The model under review builds one solid part; all positions refer to its coordinate system, in mm. A direction names the side the tool comes from. Round coordinates to 2 decimals unless told otherwise and drop trailing zeros. Answer in a Markdown table with one row per item. Add a question column.
```python
from build123d import *

# Parameters (mm, degrees)
BOSS_EXTRUDE1_DEPTH = 40
BOSS_EXTRUDE3_DEPTH = 29.899298
SKETCH3_R           = 3
CUT_EXTRUDE1_DEPTH  = 30.899298
SKETCH4_R           = 3
CUT_EXTRUDE2_DEPTH  = 38.007847
FILLET1_R           = 3
CHAMFER1_SIZE       = 1


with BuildPart() as part:
    # Sketch1 → Boss-Extrude1 (new body)
    with BuildSketch(Plane.XY):
        Polygon((0, 15), (14.899298, 15), (14.899298, -14.949649), (-15, -14.949649), (-15, 15), align=None)
        Polygon((-9.966433, 9.966433), (-4.741433, 9.966433), (-3.1, 8.307461), (-5.5, 8.307461), (-5.5, 6.667461), (-2.79, 3.957461), (2.79, 3.957461), (5.5, 6.667461), (5.5, 8.307461), (3.1, 8.307461), (4.741433, 9.966433), (9.966433, 9.966433), (9.966433, 4.741433), (8.307461, 3.1), (8.307461, 5.5), (6.667461, 5.5), (3.957461, 2.79), (3.957461, -2.79), (6.667461, -5.5), (8.307461, -5.5), (8.307461, -3.1), (9.966433, -4.741433), (9.966433, -9.966433), (4.741433, -9.966433), (3.1, -8.307461), (5.5, -8.307461), (5.5, -6.667461), (2.79, -3.957461), (-2.79, -3.957461), (-5.5, -6.667461), (-5.5, -8.307461), (-3.1, -8.307461), (-4.741433, -9.966433), (-9.966433, -9.966433), (-9.966433, -4.741433), (-8.307461, -3.1), (-8.307461, -5.5), (-6.667461, -5.5), (-3.957461, -2.79), (-3.957461, 2.79), (-6.667461, 5.5), (-8.307461, 5.5), (-8.307461, 3.1), (-9.966433, 4.741433), align=None, mode=Mode.SUBTRACT)
    extrude(amount=BOSS_EXTRUDE1_DEPTH)

    # Sketch5 → Boss-Extrude3 (add, through all)
    with BuildSketch(Plane.ZY.offset(15)):
        with BuildLine():
            Line((0, 21.5), (0, 15))
            Line((0, 15), (12, 15))
            ThreePointArc((12, 15), (9.45049, 27.47913), (16.690416, 17))
            Line((16.690416, 17), (27.804488, 17))
            Line((27.804488, 17), (40, 17))
            Line((40, 17), (40, 21))
            Line((40, 21), (23.989579, 21))
            ThreePointArc((23.989579, 21), (12.250054, 33.497394), (0, 21.5))
        make_face()
    extrude(amount=-BOSS_EXTRUDE3_DEPTH)

    # Sketch3 → Cut-Extrude1 (cut, through all)
    with BuildSketch(Plane.ZY.offset(15)):
        with Locations((12, 0)):
            Circle(SKETCH3_R)
        with Locations((27, 0)):
            Circle(SKETCH3_R)
    extrude(amount=-CUT_EXTRUDE1_DEPTH, mode=Mode.SUBTRACT)

    # Sketch4 → Cut-Extrude2 (cut, through all)
    with BuildSketch(Plane(origin=(0, 22.058198, 0), x_dir=(1, 0, 0), z_dir=(0, 1, 0))):
        with Locations((0, -32.5)):
            Circle(SKETCH4_R)
    extrude(amount=-CUT_EXTRUDE2_DEPTH, mode=Mode.SUBTRACT)

    # Fillet1
    fillet1_edges = [part.edges().sort_by_distance(p)[0] for p in [
        (-0.050351, -14.949649, 40),
        (14.899298, 0.025175, 40),
        (14.899298, 33.497394, 12.250054),
        (14.899298, 21, 31.994789),
        (14.899298, 19, 40),
        (-0.050351, 21, 40),
        (-15, 19, 40),
        (-15, 21, 31.994789),
        (-15, 33.497394, 12.250054),
        (14.899298, 0.025175, 0),
        (-0.050351, -14.949649, 0),
        (-15, 3.275175, 0),
        (-15, 0.025175, 40),
        (14.899298, -14.949649, 20),
        (-15, -14.949649, 20),
    ]]
    fillet(fillet1_edges, radius=FILLET1_R)

    # Chamfer1
    chamfer1_edges = [part.edges().sort_by_distance(p)[0] for p in [
        (14.899298, 0, 9),
        (-15, 0, 9),
        (14.899298, 0, 24),
        (-15, 0, 24),
        (-3, -14.949649, 32.5),
        (-3, 21, 32.5),
    ]]
    chamfer(chamfer1_edges, length=CHAMFER1_SIZE)


solid = part.part
```
1. Tool access review of faces 4 (the cylindrical face through (-14.14, 1.71, 39.1)), 5 (the flat face through (5.5, -7, 20)), 6 (the flat face through (0, 17, 28)): name each direction out of +Z, -Z, +X, -X, +Y, -Y from which nothing blocks a thin tool from reaching the whole face with its end or side.
2. For L1, parallel to Z at x = -11.5, y = 0; L2, parallel to Y at x = -10.5, z = 12; L3, parallel to Y at x = -6.75, z = 12, list the stretches that pass through material, from the lowest coordinate up.
3. Add section A-A on x = 0. State how many separate pieces and enclosed holes the cut face has, plus the area to 3 significant figures.
4. Mouldability with a two-part tool opening along X and no side actions: class faces 1 (the flat face through (0, 9, 0)), 2 (the cylindrical face through (-0.65, 18.52, 35.43)), 3 (the cylindrical face through (14.04, 20.1, 30.39)) as pulls with the +X half, pulls with the -X half, needs draft (parallel to the pull), parting line crosses it, or undercut.
5. Insertion check: pin 1 Ø5 at (y, z) = (22, 32.5) entering from -X; pin 2 Ø5.5 at (y, z) = (0, 27) entering from +X; pin 3 Ø5.5 at (x, z) = (-7, 21) entering from +Y; pin 4 Ø8 at (x, z) = (7.5, 9) entering from +Y. Each pin has a flat end and moves straight along its axis. Give the tip position at first contact, or say it passes through.
Filled in:
| question | item | result |
|---|---|---|
| 1 | face 4 | +Z, -X, +Y, -Y |
| 1 | face 5 | +Z, -Z |
| 1 | face 6 | +Z, +X, -X |
| 2 | L1 | 0 to 9, 15 to 24, 30 to 40 |
| 2 | L2 | -14.95 to -3, 3 to 15, 28 to 33.5 |
| 2 | L3 | -14.95 to -9.97, -5.5 to -3, 3 to 5.5, 9.97 to 15, 28 to 33.5 |
| 3 | separate pieces | 5 |
| 3 | enclosed holes | 0 |
| 3 | area | 1,010 mm² |
| 4 | face 1 | needs draft |
| 4 | face 2 | undercut |
| 4 | face 3 | pulls with the +X half |
| 5 | pin 1 | x = -14.6 |
| 5 | pin 2 | through |
| 5 | pin 3 | y = 31.74 |
| 5 | pin 4 | y = 33.5 |
